Job drawing, mm, ordinate dimensions from the low corner. One solid piece. Round coordinates to 2 decimals unless told otherwise and drop trailing zeros. Loops run counter-clockwise (first coordinate to the right, second up) from the corner with the lowest first, then second, coordinate; pieces in that order, holes last.
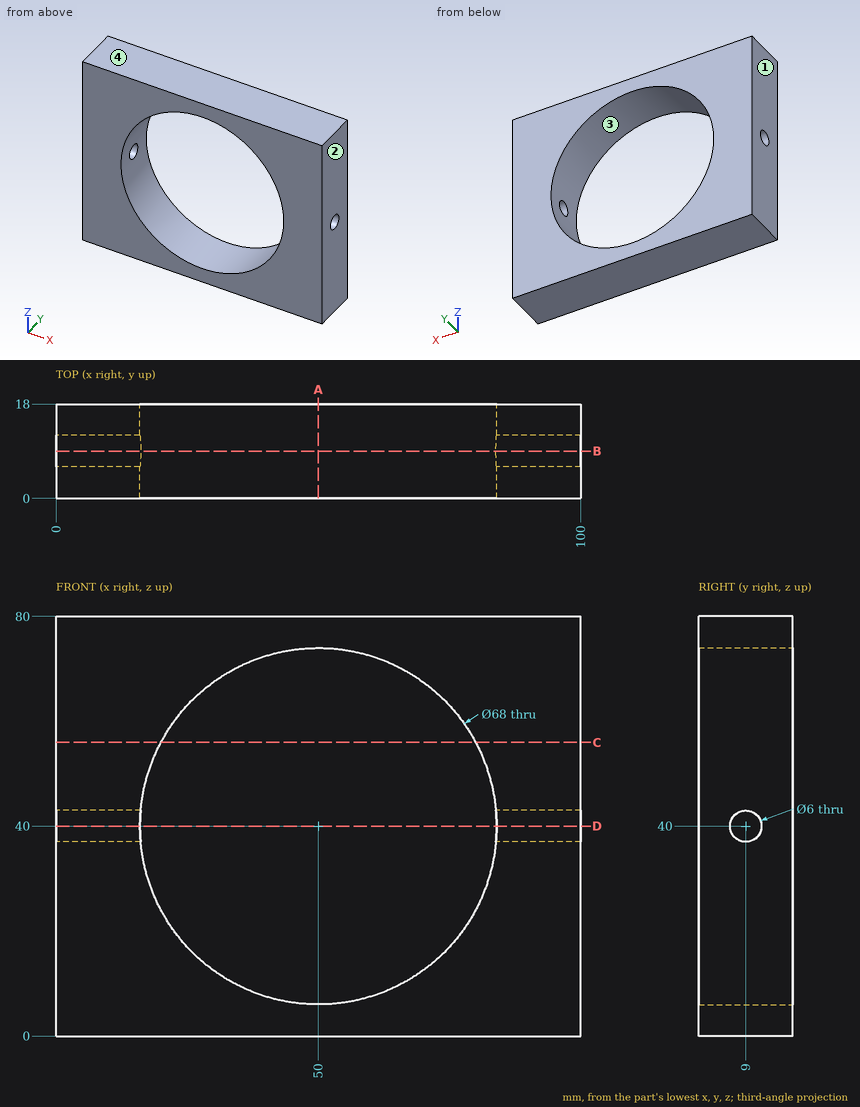
1) Mould opens along X. For the marked faces 1, 2, 3 and 4 say: released by +X, released by -X, zero draft, split by the parting line, or undercut.
Values:
face 1: released by -X
face 2: released by +X
face 3: undercut
face 4: zero draft
2) Slice it at B-B, the plane y = 9. Give the cut face in (x, z).
Values:
outline: (0, 0) - (100, 0) - (100, 37) - (83.87, 37) arc R34 cw to (16.13, 37) - (0, 37) - close; (0, 43) - (16.13, 43) arc R34 cw to (83.87, 43) - (100, 43) - (100, 80) - (0, 80) - close
3) Slice it at A-A, the plane x = 50. Give the cut face in (y, z), then the cut area to 3 significant figures.
Values:
outline: (0, 0) - (18, 0) - (18, 6) - (0, 6) - close; (0, 74) - (18, 74) - (18, 80) - (0, 80) - close
area: 216 mm2
4) Slice it at D-D, the plane z = 40. Give the cut face in (x, y).
Values:
outline: (0, 0) - (16, 0) - (16, 6) - (0, 6) - close; (0, 12) - (16, 12) - (16, 18) - (0, 18) - close; (84, 0) - (100, 0) - (100, 6) - (84, 6) - close; (84, 12) - (100, 12) - (100, 18) - (84, 18) - close
5) Wall check: line 1 along Z through (x, y) = (6, 9); line 2 along X through (y, z) = (12.5, 40); line 3 along Z through (x, y) = (50, 10.25). Give the ranges that are in metal, low to high.
Values:
line 1: z = 0 to 37, 43 to 80
line 2: x = 0 to 16, 84 to 100
line 3: z = 0 to 6, 74 to 80
6) Slice it at C-C, the plane z = 56. Give the cut face in (x, y).
Values:
outline: (0, 0) - (20, 0) - (20, 18) - (0, 18) - close; (80, 0) - (100, 0) - (100, 18) - (80, 18) - close
